Verification items for the finished model (mm, model axes). A direction names the side the tool comes from. Round coordinates to 2 decimals unless told otherwise and drop trailing zeros. Write each loop counter-clockwise with the first axis right and the second up, starting at its lowest first coordinate (ties: lowest second). Pieces come first, ordered by that corner, then holes. Notation, with made-up numbers: (-8.75, -30) - (37.25, -30) arc R21 cw to (37.25, 0) - close; hole circle Ø1 at (-20.75, -25). An arc over 180 degrees is marked (long way). Answer as a JSON object with one key per item and string values.
```python
from build123d import *

# Parameters (mm, degrees)
BOSS_EXTRUDE1_DEPTH      = 29
BOSS_EXTRUDE1_DEPTH_BACK = 29
CUT_EXTRUDE1_DEPTH       = 20
CUT_EXTRUDE1_DEPTH_BACK  = 62.202085825
SKETCH2_R                = 15
CUT_EXTRUDE2_DEPTH       = 18
SKETCH4_R                = 3
CUT_EXTRUDE3_DEPTH       = 46.847573609
CUT_EXTRUDE4_DEPTH       = 10


with BuildPart() as part:
    # Sketch1 → Boss-Extrude1 (new, two sides: drawn at the far end of the back side and taken through both)
    with BuildSketch(Plane(origin=(0, 0, 0), x_dir=(0, 0, -1), z_dir=(1, 0, 0)).offset(-BOSS_EXTRUDE1_DEPTH_BACK)):
        Polygon((-44.77382393, -30), (-25.77382393, -30), (-25.77382393, -19.08375673), (-38.27382393, -11.866878365), (-38.27382393, 2.566878365), (-25.77382393, 9.78375673), (-25.77382393, 20.15), (-44.77382393, 20.15), align=None)
    extrude(amount=BOSS_EXTRUDE1_DEPTH + BOSS_EXTRUDE1_DEPTH_BACK)

    # Sketch2 → Cut-Extrude1 (cut, two sides: drawn at the far end of the back side and taken through both)
    with BuildSketch(Plane(origin=(0, 0, 0), x_dir=(0, 0, -1), z_dir=(1, 0, 0)).offset(-CUT_EXTRUDE1_DEPTH_BACK)):
        with Locations((-25.77382393, -4.65)):
            Circle(SKETCH2_R)
    extrude(amount=CUT_EXTRUDE1_DEPTH + CUT_EXTRUDE1_DEPTH_BACK, mode=Mode.SUBTRACT)

    # Sketch3 → Cut-Extrude2 (cut)
    with BuildSketch(Plane(origin=(0, 20.15, 0), x_dir=(1, 0, 0), z_dir=(0, 1, 0))):
        with BuildLine():
            Line((9.55, -25.77382393), (1.3, -25.77382393))
            Line((1.3, -25.77382393), (1.3, -36.424528133))
            ThreePointArc((1.3, -36.424528133), (7.246263565, -32.509920723), (9.55, -25.77382393))
        make_face()
        with BuildLine():
            Line((1.3, -36.424528133), (1.3, -25.77382393))
            Line((1.3, -25.77382393), (-4.2, -25.77382393))
            Line((-4.2, -25.77382393), (-4.2, -36.424528133))
            ThreePointArc((-4.2, -36.424528133), (-1.45, -36.77382393), (1.3, -36.424528133))
        make_face()
        with BuildLine():
            Line((-4.2, -36.424528133), (-4.2, -25.77382393))
            Line((-4.2, -25.77382393), (-12.45, -25.77382393))
            ThreePointArc((-12.45, -25.77382393), (-10.146263565, -32.509920723), (-4.2, -36.424528133))
        make_face()
        with BuildLine():
            Line((1.3, -37.77382393), (1.3, -36.424528133))
            ThreePointArc((1.3, -36.424528133), (-1.45, -36.77382393), (-4.2, -36.424528133))
            Line((-4.2, -36.424528133), (-4.2, -37.77382393))
            ThreePointArc((-4.2, -37.77382393), (-3.907106781, -38.480930712), (-3.2, -38.77382393))
            Line((-3.2, -38.77382393), (0.3, -38.77382393))
            ThreePointArc((0.3, -38.77382393), (1.007106781, -38.480930712), (1.3, -37.77382393))
        make_face()
    extrude(amount=-CUT_EXTRUDE2_DEPTH, mode=Mode.SUBTRACT)

    # Sketch4 → Cut-Extrude3 (cut, through all)
    with BuildSketch(Plane(origin=(0, 0, 25.77382393), x_dir=(-1, 0, 0), z_dir=(0, 0, -1))):
        with Locations((-22, 15.255553499)):
            Circle(SKETCH4_R)
        with Locations((-22, -25.105553499)):
            Circle(SKETCH4_R)
        with Locations((22, -25.105553499)):
            Circle(SKETCH4_R)
        with Locations((22, 15.255553499)):
            Circle(SKETCH4_R)
    extrude(amount=-CUT_EXTRUDE3_DEPTH, mode=Mode.SUBTRACT)

    # Sketch5 → Cut-Extrude4 (cut)
    with BuildSketch(Plane.XY.offset(44.77382393)):
        Polygon((-19.834936491, -21.355553499), (-24.165063509, -21.355553499), (-26.330127019, -25.105553499), (-24.165063509, -28.855553499), (-19.834936491, -28.855553499), (-17.669872981, -25.105553499), align=None)
        Polygon((-19.834936491, 11.505553499), (-17.669872981, 15.255553499), (-19.834936491, 19.005553499), (-24.165063509, 19.005553499), (-26.330127019, 15.255553499), (-24.165063509, 11.505553499), align=None)
        Polygon((17.669872981, 15.255553499), (19.834936491, 11.505553499), (24.165063509, 11.505553499), (26.330127019, 15.255553499), (24.165063509, 19.005553499), (19.834936491, 19.005553499), align=None)
        Polygon((24.165063509, -21.355553499), (19.834936491, -21.355553499), (17.669872981, -25.105553499), (19.834936491, -28.855553499), (24.165063509, -28.855553499), (26.330127019, -25.105553499), align=None)
    extrude(amount=-CUT_EXTRUDE4_DEPTH, mode=Mode.SUBTRACT)


solid = part.part
```
Q1. Section check A-A, the plane x = 22. Record the cut outline in (y, z), then the cut area to 3 significant figures.
Geometry check:
{"outline": "(-30, 25.77) - (-28.11, 25.77) - (-28.11, 34.77) - (-28.86, 34.77) - (-28.86, 44.77) - (-30, 44.77) - close; (-22.11, 25.77) - (-19.08, 25.77) - (-11.87, 38.27) - (2.57, 38.27) - (9.78, 25.77) - (12.26, 25.77) - (12.26, 34.77) - (11.51, 34.77) - (11.51, 44.77) - (-21.36, 44.77) - (-21.36, 34.77) - (-22.11, 34.77) - close; (18.26, 25.77) - (20.15, 25.77) - (20.15, 44.77) - (19.01, 44.77) - (19.01, 34.77) - (18.26, 34.77) - close", "area": "424 mm2"}
Q2. Set-up check for faces 1 (the cylindrical face through (-4.84, -4.32, 40.77)), 2 (the flat face through (-25.23, -23.2, 39.84)), 3 (the flat face through (-4.2, 12, 37)), 4 (the cylindrical face through (24.38, -26.93, 30.21)): record each of +Z, -Z, +X, -X, +Y, -Y from which the full face is reachable in a straight line by a thin tool's end or side.
Geometry check:
{"face 1": "-Z, -X", "face 2": "+Z", "face 3": "-Z, +Y", "face 4": "+Z, -Z"}
Q3. Section check C-C, the plane x = -22. Record the cut outline in (y, z), then the cut area to 3 significant figures.
Geometry check:
{"outline": "(-30, 25.77) - (-28.11, 25.77) - (-28.11, 34.77) - (-28.86, 34.77) - (-28.86, 44.77) - (-30, 44.77) - close; (-22.11, 25.77) - (-19.65, 25.77) arc R15 cw to (10.35, 25.77) - (12.26, 25.77) - (12.26, 34.77) - (11.51, 34.77) - (11.51, 44.77) - (-21.36, 44.77) - (-21.36, 34.77) - (-22.11, 34.77) - close; (18.26, 25.77) - (20.15, 25.77) - (20.15, 44.77) - (19.01, 44.77) - (19.01, 34.77) - (18.26, 34.77) - close", "area": "341 mm2"}
Q4. Section check B-B, the plane y = -24. Record the cut outline in (x, z).
Geometry check:
{"outline": "(-29, 25.77) - (-24.79, 25.77) - (-24.79, 34.77) - (-25.69, 34.77) - (-25.69, 44.77) - (-29, 44.77) - close; (-19.21, 25.77) - (19.21, 25.77) - (19.21, 34.77) - (18.31, 34.77) - (18.31, 44.77) - (-18.31, 44.77) - (-18.31, 34.77) - (-19.21, 34.77) - close; (24.79, 25.77) - (29, 25.77) - (29, 44.77) - (25.69, 44.77) - (25.69, 34.77) - (24.79, 34.77) - close"}
Q5. Release check for a two-part mould opening along X. For faces 5 (the flat face through (20, -5, 39)), 6 (the flat face through (29, -5, 40)), 7 (the flat face through (-25.263, 13.407, 39.844)), 8 (the flat face through (24.437, 6.125, 32.111)) record: released by +X, released by -X, zero draft, split by the parting line, or undercut.
Geometry check:
{"face 5": "released by -X", "face 6": "released by +X", "face 7": "undercut", "face 8": "zero draft"}
Q6. Material ranges on line 1 along Y through (x, z) = (22, 28.25); line 2 along Y through (x, z) = (24.5, 41.25); line 3 along Y through (x, z) = (23.5, 35.5), recorded low to high. Write a range as [from, to].
Geometry check:
{"line 1": "y = [-30, -28.11], [-22.11, -17.65], [8.35, 12.26], [18.26, 20.15]", "line 2": "y = [-30, -28.28], [-21.94, 12.09], [18.43, 20.15]", "line 3": "y = [-30, -28.86], [-21.36, -13.47], [4.17, 11.51], [19.01, 20.15]"}
Q7. Gauge pin test, flat end, axial feed: P1, Ø4, axis at x = -21.5, y = -23.5, coming from the +Z side. Record the tip position at first contact, or that the pin passes through.
Geometry check:
{"P1": "stops at z = 34.77"}
Q8. Section check D-D, the plane z = 35.5. State how many separate pieces and enclosed holes the cut face has, then the cut area to 3 significant figures.
Geometry check:
{"separate pieces": "3", "enclosed holes": "4", "area": "1,300 mm2"}
